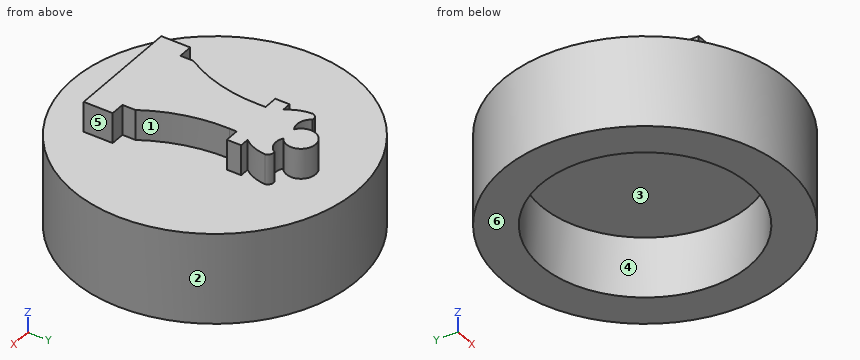
from build123d import *

# Parameters (mm, degrees)
SKETCH1_R           = 11.938
SKETCH1_R_2         = 8.763
BOSS_EXTRUDE1_DEPTH = 5.08
SKETCH2_R           = 11.938
BOSS_EXTRUDE2_DEPTH = 2.54
BOSS_EXTRUDE7_DEPTH = 2.54


with BuildPart() as part:
    # Sketch1 → Boss-Extrude1 (new body)
    with BuildSketch(Plane.XY):
        Circle(SKETCH1_R)
        Circle(SKETCH1_R_2, mode=Mode.SUBTRACT)
    extrude(amount=BOSS_EXTRUDE1_DEPTH)

    # Sketch2 → Boss-Extrude2 (add)
    with BuildSketch(Plane.XY.offset(5.08)):
        Circle(SKETCH2_R)
    extrude(amount=BOSS_EXTRUDE2_DEPTH)

    # Sketch3 → Boss-Extrude7 (add)
    with BuildSketch(Plane.XY.offset(7.62)):
        with BuildLine():
            Line((-3.581203205, -5.323066216), (-3.581203205, -4.234628776))
            ThreePointArc((-3.581203205, -4.234628776), (-2.206146934, -1.034066779), (-1.780332767, 2.423252867))
            Line((-1.780332767, 2.423252867), (-1.780332767, 3.033045049))
            Line((-1.780332767, 3.033045049), (-2.98662319, 3.033045049))
            Line((-2.98662319, 3.033045049), (-2.98662319, 4.229885576))
            Line((-2.98662319, 4.229885576), (-2.200089182, 4.229885576))
            ThreePointArc((-2.200089182, 4.229885576), (-2.736363422, 5.164361527), (-2.950097006, 6.220369728))
            ThreePointArc((-2.950097006, 6.220369728), (-2.730043081, 6.525801031), (-2.358468914, 6.586171955))
            ThreePointArc((-2.358468914, 6.586171955), (-1.595642249, 6.036578644), (-0.667621184, 6.187357394))
            ThreePointArc((-0.667621184, 6.187357394), (0, 8.443971822), (0.667621184, 6.187357394))
            ThreePointArc((0.667621184, 6.187357394), (1.595642249, 6.036578644), (2.358468914, 6.586171955))
            ThreePointArc((2.358468914, 6.586171955), (2.730043081, 6.525801031), (2.950097006, 6.220369728))
            ThreePointArc((2.950097006, 6.220369728), (2.736363422, 5.164361527), (2.200089182, 4.229885576))
            Line((2.200089182, 4.229885576), (2.98662319, 4.229885576))
            Line((2.98662319, 4.229885576), (2.98662319, 3.033045049))
            Line((2.98662319, 3.033045049), (1.780332767, 3.033045049))
            Line((1.780332767, 3.033045049), (1.780332767, 2.423252867))
            ThreePointArc((1.780332767, 2.423252867), (2.206146934, -1.034066779), (3.581203205, -4.234628776))
            Line((3.581203205, -4.234628776), (3.581203205, -5.323066216))
            Line((3.581203205, -5.323066216), (4.782890844, -5.323066216))
            Line((4.782890844, -5.323066216), (4.782890844, -7.750587613))
            Line((4.782890844, -7.750587613), (-4.798911093, -7.750587613))
            Line((-4.798911093, -7.750587613), (-4.798911093, -5.323066216))
            Line((-4.798911093, -5.323066216), (-3.581203205, -5.323066216))
        make_face()
    extrude(amount=BOSS_EXTRUDE7_DEPTH)


solid = part.part
Here's how the part is built. I have some questions about the finished solid (model axes, mm). Face numbers are marked on the shaded views. A direction names the side the tool comes from. Coordinates: 2 decimals unless noted, no trailing zeros. Order: outer loops, then holes, each group sorted by start corner. A loop starts at its lowest first (then second) coordinate and runs counter-clockwise, first axis right, second up. Notation, with made-up numbers: M -35.5,-2 L 16.5,-2 A33 ccw 16.5,26 Z; hole C -39.5,3.25 d4. An arc over 180 degrees is marked long. Answer as CSV lines item,"result".
Item 1: For pin 1 (3 mm diameter, centred on y = 8.5, z = 6, fed in from +X); pin 2 (0.7 mm diameter, centred on y = 2.5, z = 9.5, fed in from +X); pin 3 (0.6 mm diameter, centred on x = -3, z = 8.5, fed in from +Y), each with a flat end and sliding along its axis, tell me the tip position at first contact or that it passes through.
Results found:
pin 1,"x = 9.67"
pin 2,"x = 1.78"
pin 3,"y = 6.54"
Item 2: Imagine slicing it at B-B on y = 0. Write out the boundary of the cut face in (x, z), plus the area to 3 significant figures.
Results found:
outline,"M -11.94,0 L -8.76,0 L -8.76,5.08 L 8.76,5.08 L 8.76,0 L 11.94,0 L 11.94,7.62 L 1.97,7.62 L 1.97,10.16 L -1.97,10.16 L -1.97,7.62 L -11.94,7.62 Z"
area,"103 mm2"
Item 3: Imagine slicing it at C-C on x = 6.25. Write out the boundary of the cut face in (y, z).
Results found:
outline,"M -10.17,0 L -6.14,0 L -6.14,5.08 L 6.14,5.08 L 6.14,0 L 10.17,0 L 10.17,7.62 L -10.17,7.62 Z"
Item 4: Imagine slicing it at D-D on y = 10.75. Write out the boundary of the cut face in (x, z).
Results found:
outline,"M -5.19,0 L 5.19,0 L 5.19,7.62 L -5.19,7.62 Z"
Item 5: We'd pull the mould along X, two halves only. Please class the marked faces 4, 5 and 6: +X half, -X half, draft (parallel to the pull), parting line (faces both ways), or undercut.
Results found:
face 4,"undercut"
face 5,"+X half"
face 6,"draft"
Item 6: If I drill on line 1 (Y direction, x = 0, z = 3.75); line 2 (Z direction, x = -4, y = 1.5); line 3 (Z direction, x = -0.75, y = 1), over which ranges is the centre line in solid material (lowest first)?
Results found:
line 1,"-11.94 to -8.76, 8.76 to 11.94"
line 2,"5.08 to 7.62"
line 3,"5.08 to 10.16"
Item 7: Imagine slicing it at A-A on x = 0. Write out the boundary of the cut face in (y, z), plus the area to 3 significant figures.
Results found:
outline,"M -11.94,0 L -8.76,0 L -8.76,5.08 L 8.76,5.08 L 8.76,0 L 11.94,0 L 11.94,7.62 L 8.44,7.62 L 8.44,10.16 L -7.75,10.16 L -7.75,7.62 L -11.94,7.62 Z"
area,"134 mm2"
Item 8: On a 3-axis mill with a long thin cutter (end or side, diameter ignored), from which of +Z, -Z, +X, -X, +Y, -Y can I reach the whole of each face in a straight line? I mean the marked faces 1, 2 and 3. Say none if no direction works.
Results found:
face 1,"+Z, +X"
face 2,"+Z, -Z"
face 3,"-Z"
